from build123d import *

# Parameters (mm, degrees)
SKETCH1_R           = 2
BOSS_EXTRUDE1_DEPTH = 370
SKETCH2_R           = 2
CUT_EXTRUDE1_DEPTH  = 27
SKETCH3_R           = 2
CUT_EXTRUDE2_DEPTH  = 28


with BuildPart() as part:
    # Sketch1 → Boss-Extrude1 (new body)
    with BuildSketch(Plane.XY):
        Polygon((-10, -10), (-3.5, -10), (-3.5, -9), (-3, -9), (-3, -8), (-5.5, -8), (-5.5, -6.560660172), (-3.44, -4.500660172), (3.44, -4.500660172), (5.5, -6.560660172), (5.5, -8), (3, -8), (3, -9), (3.5, -9), (3.5, -10), (10, -10), (10, -3.5), (9, -3.5), (9, -3), (8, -3), (8, -5.5), (6.560660172, -5.5), (4.500660172, -3.44), (4.500660172, 3.44), (6.560660172, 5.5), (8, 5.5), (8, 3), (9, 3), (9, 3.5), (10, 3.5), (10, 10), (3.5, 10), (3.5, 9), (3, 9), (3, 8), (5.5, 8), (5.5, 6.560660172), (3.44, 4.500660172), (-3.44, 4.500660172), (-5.5, 6.560660172), (-5.5, 8), (-3, 8), (-3, 9), (-3.5, 9), (-3.5, 10), (-10, 10), (-10, 3.5), (-9, 3.5), (-9, 3), (-8, 3), (-8, 5.5), (-6.560660172, 5.5), (-4.500660172, 3.44), (-4.500660172, -3.44), (-6.560660172, -5.5), (-8, -5.5), (-8, -3), (-9, -3), (-9, -3.5), (-10, -3.5), align=None)
        Circle(SKETCH1_R, mode=Mode.SUBTRACT)
    extrude(amount=BOSS_EXTRUDE1_DEPTH)

    # Sketch2 → Cut-Extrude1 (cut)
    with BuildSketch(Plane(origin=(0, 10, 0), x_dir=(1, 0, 0), z_dir=(0, 1, 0))):
        with Locations(Location((0, -15, 0), (0, 0, 270))):
            Circle(SKETCH2_R)
        with Locations(Location((0, -30, 0), (0, 0, 270))):
            Circle(SKETCH2_R)
        with Locations(Location((0, -355, 0), (0, 0, 270))):
            Circle(SKETCH2_R)
        with Locations(Location((0, -340, 0), (0, 0, 270))):
            Circle(SKETCH2_R)
    extrude(amount=-CUT_EXTRUDE1_DEPTH, mode=Mode.SUBTRACT)

    # Sketch3 → Cut-Extrude2 (cut)
    with BuildSketch(Plane.XZ.offset(4.500660172)):
        with Locations(Location((0, 80, 0), (0, 0, 270))):
            Circle(SKETCH3_R)
        with Locations(Location((0, 290, 0), (0, 0, 270))):
            Circle(SKETCH3_R)
    extrude(amount=-CUT_EXTRUDE2_DEPTH, mode=Mode.SUBTRACT)


solid = part.part
For this review, take the finished solid that the model builds, in its own axes (mm). A direction names the side the tool comes from. Give positions to 0.01 mm unless a question says otherwise; leave off trailing zeros. Use CSV: the item, a comma, the result in double quotes.
Q1. For P1, Ø3.5, axis at x = 0, y = 0, coming from the +Z side; P2, Ø4, axis at x = -1.5, y = -2, coming from the -Z side; P3, Ø6.5, axis at x = 0, z = 15, coming from the -Y side; P4, Ø6.5, axis at x = 0, z = 340, coming from the +Y side, all flat-tipped, find the tip position at first contact; note any pin that passes through.
Conclusion:
P1,"through"
P2,"z = 0"
P3,"y = -9"
P4,"y = 9"
Q2. Tool access review of faces 4 (the face through (7, 10, 182)), 5 (the face through (0, -4.501, 182)): name each direction out of +Z, -Z, +X, -X, +Y, -Y from which nothing blocks a thin tool from reaching the whole face with its end or side.
Conclusion:
face 4,"+Z, -Z, +X, -X, +Y"
face 5,"+Z, -Z"
Q3. To check wall thickness, follow probe 1 along Y at (x, z) = (-3.25, 153); probe 2 along X at (y, z) = (0, 9); probe 3 along X at (y, z) = (3.2, 290). State the ranges of each line that lie inside material, in increasing order. Write a range as [from, to].
Conclusion:
probe 1,"[-9, -8], [-4.5, 4.5], [8, 9]"
probe 2,"[-4.5, -2], [2, 4.5]"
probe 3,"[-9, -8], [-4.5, -2], [2, 4.5], [8, 9]"
Q4. Mouldability with a two-part tool opening along Y and no side actions: class faces 1 (the face through (10, 7, 182)), 2 (the face through (0, 4.501, 182)), 3 (the face through (-7, 10, 182)) as pulls with the +Y half, pulls with the -Y half, needs draft (parallel to the pull), parting line crosses it, or undercut.
Conclusion:
face 1,"needs draft"
face 2,"undercut"
face 3,"pulls with the +Y half"
